Drawing for the job (mm, zero at the part's lowest x, y, z). A direction names the side the tool comes from. Give positions to 0.01 mm unless a question says otherwise; leave off trailing zeros. Order: outer loops, then holes, each group sorted by start corner. A loop starts at its lowest first (then second) coordinate and runs counter-clockwise, first axis right, second up. Notation, with made-up numbers: (-39.5, 77) - (15.5, 77) arc R10 ccw to (15.5, 93) - close; hole circle Ø10 at (29, -37.5). An arc over 180 degrees is marked (long way). One line per item, written item: value.
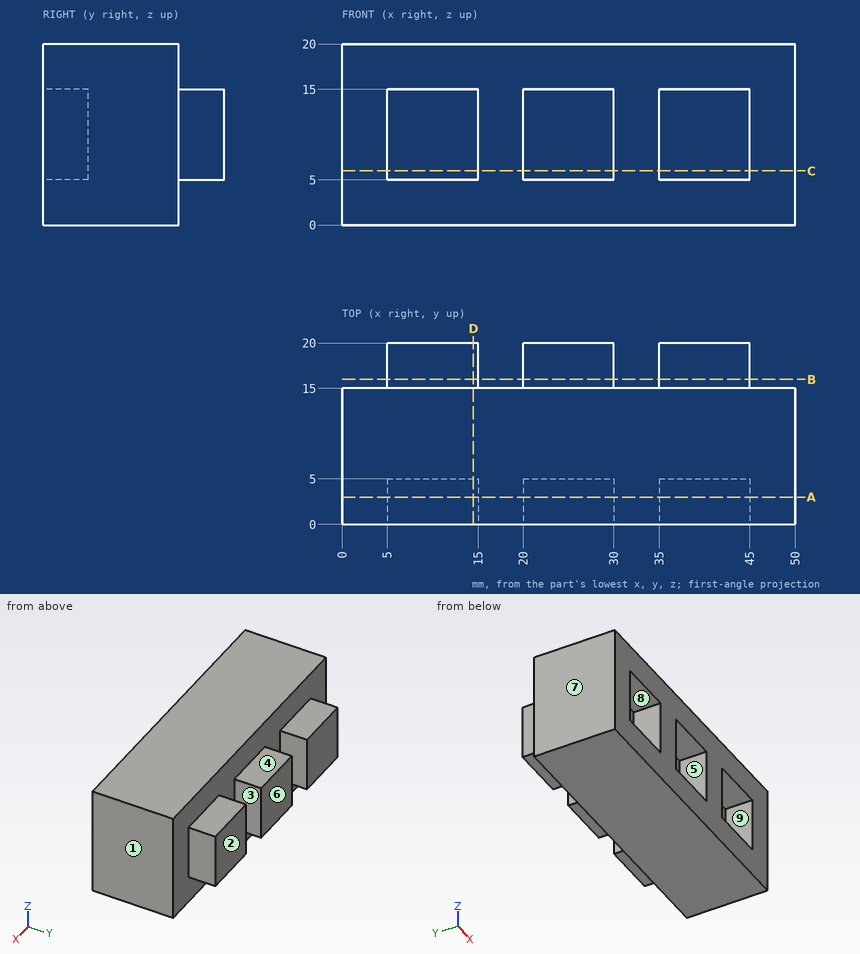
(1) Drill centre lines: line 1 (X direction, y = 1, z = 11); line 2 (Z direction, x = 13.5, y = 1.5); line 3 (Y direction, x = 32.5, z = 8.25). Where is each one in solid material? Low to high.
Completed:
line 1: 0 to 5, 15 to 20, 30 to 35, 45 to 50
line 2: 0 to 5, 15 to 20
line 3: 0 to 15
(2) Slice it at C-C, the plane z = 6. Give the cut face in (x, y), and give its area (3 significant figures).
Completed:
outline: (0, 0) - (5, 0) - (5, 5) - (15, 5) - (15, 0) - (20, 0) - (20, 5) - (30, 5) - (30, 0) - (35, 0) - (35, 5) - (45, 5) - (45, 0) - (50, 0) - (50, 15) - (45, 15) - (45, 20) - (35, 20) - (35, 15) - (30, 15) - (30, 20) - (20, 20) - (20, 15) - (15, 15) - (15, 20) - (5, 20) - (5, 15) - (0, 15) - close
area: 750 mm²
(3) Pull direction X, two halves, no side cores. Call the marked faces 6, 7, 8 and 9: +X half, -X half, draft (parallel to the pull), parting line (faces both ways), or undercut.
Completed:
face 6: draft
face 7: -X half
face 8: undercut
face 9: undercut
(4) Slice it at A-A, the plane y = 3. Give the cut face in (x, z), and give its area (3 significant figures).
Completed:
outline: (0, 0) - (50, 0) - (50, 20) - (0, 20) - close; hole (5, 5) - (15, 5) - (15, 15) - (5, 15) - close; hole (20, 5) - (30, 5) - (30, 15) - (20, 15) - close; hole (35, 5) - (45, 5) - (45, 15) - (35, 15) - close
area: 700 mm²
(5) Slice it at B-B, the plane y = 16. Give the cut face in (x, z), and give its area (3 significant figures).
Completed:
outline: (5, 5) - (15, 5) - (15, 15) - (5, 15) - close; (20, 5) - (30, 5) - (30, 15) - (20, 15) - close; (35, 5) - (45, 5) - (45, 15) - (35, 15) - close
area: 300 mm²
(6) Slice it at D-D, the plane x = 14.5. Give the cut face in (y, z).
Completed:
outline: (0, 0) - (15, 0) - (15, 5) - (20, 5) - (20, 15) - (15, 15) - (15, 20) - (0, 20) - (0, 15) - (5, 15) - (5, 5) - (0, 5) - close
(7) Pin check, flat tips, straight feed: P1, Ø1, axis at x = 26, z = 7, coming from the -Y side; P2, Ø2.5, axis at y = 17, z = 7.5, coming from the -X side; P3, Ø5.5, axis at x = 40, y = 18, coming from the +Z side. Stop position of each tip, or through.
Completed:
P1: y = 5
P2: x = 5
P3: z = 15
(8) 3-axis set-ups, long thin cutter, end or side, ignore diameter. For the marked faces 1, 2, 3, 4 and 5: which of +Z, -Z, +X, -X, +Y, -Y reach the whole face in a straight line?
Completed:
face 1: +Z, -Z, +X, +Y, -Y
face 2: +Z, -Z, +X, -X, +Y
face 3: +Z, -Z, +Y
face 4: +Z, +X, -X, +Y
face 5: -Y
